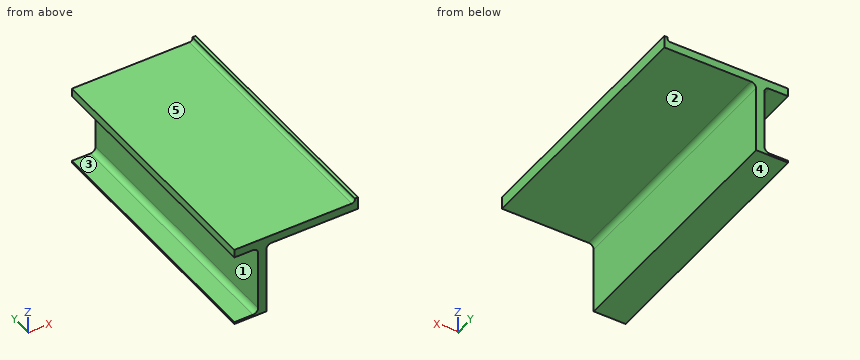
```python
from build123d import *

# Parameters (mm, degrees)
PAD_DEPTH   = 250
FILLET_R    = 5
FILLET001_R = 5
FILLET002_R = 5
FILLET003_R = 3


with BuildPart() as part:
    # Sketch → Pad (new body)
    with BuildSketch(Plane.XZ):
        Polygon((57, 77), (-60, 77), (-60, 69), (-37, 69), (-37, 1), (-60, 1), (-60, -1), (-37, -1), (-29, -1), (-29, 69), (60, 69), (60, 77), (60, 81), (57, 81), align=None)
    extrude(amount=PAD_DEPTH)

    # Fillet
    fillet_edges = [part.edges().sort_by_distance(p)[0] for p in [
        (-29, -125, 69),
    ]]
    fillet(fillet_edges, radius=FILLET_R)

    # Fillet001
    fillet001_edges = [part.edges().sort_by_distance(p)[0] for p in [
        (-37, -125, 69),
    ]]
    fillet(fillet001_edges, radius=FILLET001_R)

    # Fillet002
    fillet002_edges = [part.edges().sort_by_distance(p)[0] for p in [
        (-37, -125, 1),
    ]]
    fillet(fillet002_edges, radius=FILLET002_R)

    # Fillet003
    fillet003_edges = [part.edges().sort_by_distance(p)[0] for p in [
        (57, -125, 77),
    ]]
    fillet(fillet003_edges, radius=FILLET003_R)


solid = part.part
```
Could you check a few things on this model? Use its own coordinates, in mm. Face numbers are marked on the shaded views. A direction names the side the tool comes from. Round coordinates to 2 decimals unless told otherwise and drop trailing zeros. Write each loop counter-clockwise with the first axis right and the second up, starting at its lowest first coordinate (ties: lowest second). Pieces come first, ordered by that corner, then holes. Notation, with made-up numbers: M 16.5,-22 L 48.5,-22 A34 ccw 48.5,10 Z; hole C -25,36 d11. An arc over 180 degrees is marked long. Answer in a Markdown table with one row per item. Add a question column.
Q1. Imagine slicing it at C-C (x = -3). Please give me the cut outline in (y, z), then the cut area to 3 significant figures.
Q2. If we mould it in two halves opening along Z, with no side actions, what happens to the marked faces 3, 4 and 5? For each: +Z half, -Z half, draft (parallel to the pull), parting line (faces both ways), or undercut.
Q3. On a 3-axis mill with a long thin cutter (end or side, diameter ignored), from which of +Z, -Z, +X, -X, +Y, -Y can I reach the whole of each face in a straight line? I mean the marked faces 1 and 2. Say none if no direction works.
Q4. If I drill on line 1 (Z direction, x = -51.5, y = -171); line 2 (X direction, y = -239, z = 19); line 3 (Z direction, x = -10, y = -116), over which ranges is the centre line in solid material (lowest first)? Write a range as from..to.
Q5. Imagine slicing it at A-A (y = -48). Please give me the cut outline in (x, z).
Q6. Will these pins go through, and if not, where does the flat tip stop? pin 1 Ø0.8 at (y, z) = (-94, 80.5) entering from -X; pin 2 Ø2 at (y, z) = (-112, 41.5) entering from -X; pin 3 Ø19.5 at (y, z) = (-157, 21) entering from +X.
Q7. Imagine slicing it at B-B (z = 36). Please give me the cut outline in (x, y), then the cut area to 3 significant figures.
Values:
| question | item | result |
|---|---|---|
| 1 | outline | M -250,69 L 0,69 L 0,77 L -250,77 Z |
| 1 | area | 2,000 mm^2 |
| 2 | face 3 | undercut |
| 2 | face 4 | -Z half |
| 2 | face 5 | +Z half |
| 3 | face 1 | -X, +Y, -Y |
| 3 | face 2 | -Z, +X, +Y, -Y |
| 4 | line 1 | -1..1, 69..77 |
| 4 | line 2 | -37..-29 |
| 4 | line 3 | 69..77 |
| 5 | outline | M -60,-1 L -29,-1 L -29,64 A5 cw -24,69 L 60,69 L 60,81 L 57,81 L 57,80 A3 cw 54,77 L -60,77 L -60,69 L -42,69 A5 cw -37,64 L -37,6 A5 cw -42,1 L -60,1 Z |
| 6 | pin 1 | x = 57 |
| 6 | pin 2 | x = -37 |
| 6 | pin 3 | x = -29 |
| 7 | outline | M -37,-250 L -29,-250 L -29,0 L -37,0 Z |
| 7 | area | 2,000 mm^2 |
